Check sheet for the drawn part. Datum: minimum x, y, z corner. Units: mm. Coordinates: 2 decimals unless noted, no trailing zeros. Write each loop counter-clockwise with the first axis right and the second up, starting at its lowest first coordinate (ties: lowest second). Pieces come first, ordered by that corner, then holes. Notation, with made-up numbers: (46, 14.5) - (93, 14.5) arc R19 ccw to (93, 44.5) - close; hole circle Ø10 at (-27.75, 74.25). An arc over 180 degrees is marked (long way). Use CSV: the item, a comma, the result in double quotes. Start each with the question number.
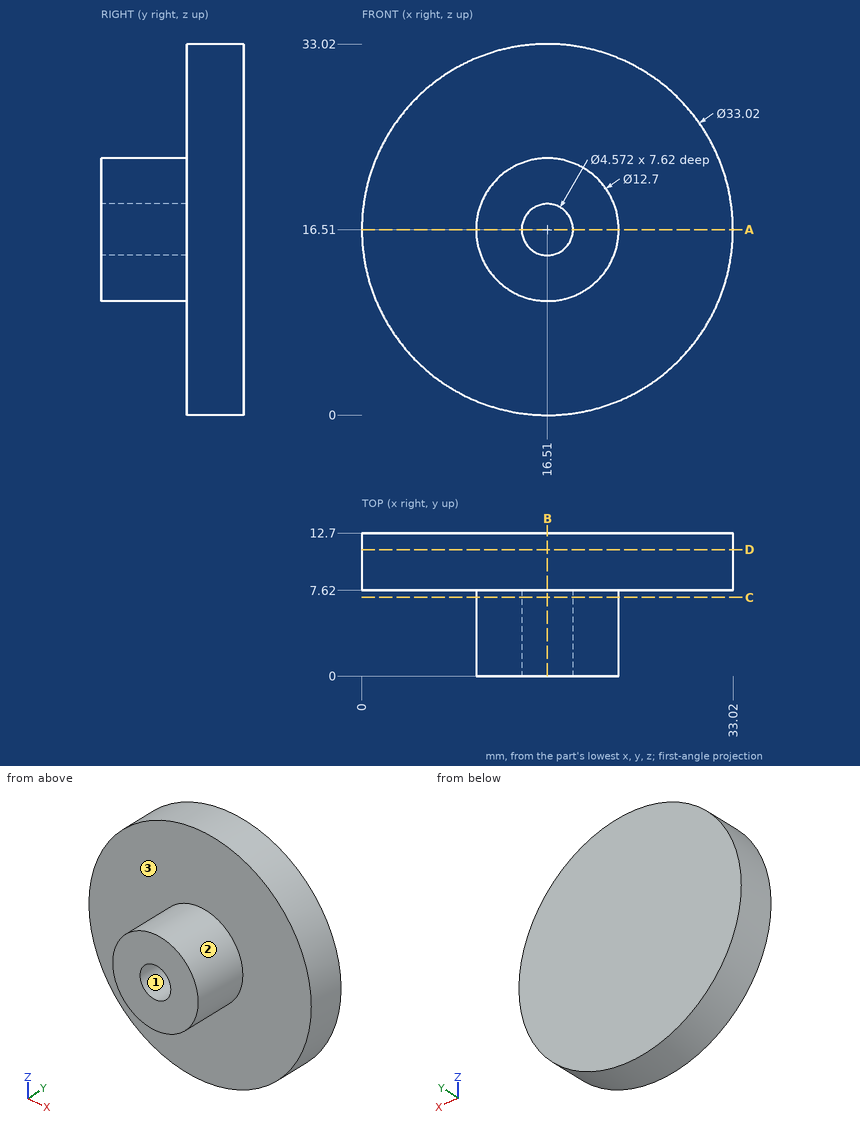
Q1. Cross-section at A-A (z = 16.51). Record the cut outline in (x, y).
Q2. Gauge pin test, flat ends, axial feed: pin 1 (3 mm diameter, centred on y = 8, z = 6, fed in from -X); pin 2 (1.5 mm diameter, centred on x = 29.5, y = 9, fed in from -Z); pin 3 (5 mm diameter, centred on y = 7.5, z = 13.5, fed in from +X). Record the tip position at first contact, or that the pin passes through.
Q3. Release check for a two-part mould opening along Z. For the marked faces 1, 2 and 3 record: released by +Z, released by -Z, zero draft, split by the parting line, or undercut.
Q4. Cross-section at B-B (x = 16.51). Record the cut outline in (y, z), plus the area to 3 significant figures.
Q5. Cross-section at D-D (y = 11.25). Record the cut outline in (x, z).
Q6. Scan lines: line 1 along Z through (x, y) = (16.51, 3.75); line 2 along Y through (x, z) = (16, 8); line 3 along Z through (x, y) = (16, 4). Record each from-to range of solid material in increasing order. Write a range as from..to.
Q7. Cross-section at C-C (y = 7). Record the cut outline in (x, z).
Reply:
1,outline,"(0, 7.62) - (10.16, 7.62) - (10.16, 0) - (14.22, 0) - (14.22, 7.62) - (18.8, 7.62) - (18.8, 0) - (22.86, 0) - (22.86, 7.62) - (33.02, 7.62) - (33.02, 12.7) - (0, 12.7) - close"
2,pin 1,"x = 2.68"
2,pin 2,"z = 5.43"
2,pin 3,"x = 33.01"
3,face 1,"undercut"
3,face 2,"split by the parting line"
3,face 3,"zero draft"
4,outline,"(0, 10.16) - (7.62, 10.16) - (7.62, 0) - (12.7, 0) - (12.7, 33.02) - (7.62, 33.02) - (7.62, 22.86) - (0, 22.86) - (0, 18.8) - (7.62, 18.8) - (7.62, 14.22) - (0, 14.22) - close"
4,area,"230 mm^2"
5,outline,"circle Ø33.02 at (16.51, 16.51)"
6,line 1,"10.16..14.22, 18.8..22.86"
6,line 2,"7.62..12.7"
6,line 3,"10.18..14.28, 18.74..22.84"
7,outline,"circle Ø12.7 at (16.51, 16.51); hole circle Ø4.57 at (16.51, 16.51)"
